Check sheet for the modelled part. Datum: model origin and axes. Units: mm. A direction names the side the tool comes from. Round coordinates to 2 decimals unless told otherwise and drop trailing zeros. Write each loop counter-clockwise with the first axis right and the second up, starting at its lowest first coordinate (ties: lowest second). Pieces come first, ordered by that corner, then holes. Notation, with made-up numbers: (-25.75, 3) -> (31.25, 3) arc R18 ccw to (31.25, 8) -> close; hole circle Ø6 at (53.5, 32). An arc over 180 degrees is marked (long way). Use one line per item in the form item = value. Start each with the question number.
```python
from build123d import *

# Parameters (mm, degrees)
F2_R = 2


with BuildPart() as f1:
    # F0 (on Right) → F1 (revolve)
    with BuildSketch(Plane.YZ):
        Polygon((0, 22), (0, 6), (48.5, 6), (48.5, 15), (48, 15), (48, 30), (8.5, 30), (8.5, 18), (6.5, 18), (6.5, 22), align=None)
    revolve(axis=Axis((0, 19.820221, 0), (0, 1, 0)))

    # F2
    f2_edges = [f1.edges().sort_by_distance(p)[0] for p in [
        (0, 0, -22),
        (0, 8.5, -30),
        (0, 48, -30),
    ]]
    fillet(f2_edges, radius=F2_R)


solid = f1.part
```
1. Sectioned sample at B-B (z = 0). Enter the section's corners in (x, y).
2. Scan lines: probe 1 along Y at (x, z) = (-5.5, -18); probe 2 along X at (y, z) = (36, 0); probe 3 along Y at (x, z) = (23, -13). Record each from-to range of solid material in increasing order.
3. Sectioned sample at A-A (x = 0). Enter the section's corners in (y, z).
4. Depth check by flat-ended pin: pin 1 (4 mm diameter, centred on y = 12.5, z = 15, fed in from +X); pin 2 (3 mm diameter, centred on x = 10, y = 40, fed in from -Z); pin 3 (2 mm diameter, centred on y = 8, z = 19, fed in from +X). Enter the tip coordinate at first touch or a pass-through.
5. Mould release check, pull along Y, two halves, no side actions. Record for faces 1 (the face through (-6.5, 48.5, 0.2)), 2 (the face through (-16.2, 6.5, 8.3)), 3 (the face through (-21.477, 4.219, -4.769)): +Y half, -Y half, draft (parallel to the pull), parting line (faces both ways), or undercut.
6. Sectioned sample at C-C (y = 29). Enter the section's corners in (x, z), and give its area (3 significant figures).
7. Tool access check on faces 4 (the face through (0, 25, -6)), 5 (the face through (0.66, 48.246, -14.985)), 6 (the face through (17.847, 7.486, -2.343)). Record the directions out of +Z, -Z, +X, -X, +Y, -Y that give a thin tool (end or side, any length) a straight path to the whole face; none if there is none.
Returned:
q1.outline = (-30, 10.5) arc R2 ccw to (-28, 8.5) -> (-18, 8.5) -> (-18, 6.5) -> (-22, 6.5) -> (-22, 2) arc R2 ccw to (-20, 0) -> (-6, 0) -> (-6, 48.5) -> (-15, 48.5) -> (-15, 48) -> (-28, 48) arc R2 ccw to (-30, 46) -> close; (6, 0) -> (20, 0) arc R2 ccw to (22, 2) -> (22, 6.5) -> (18, 6.5) -> (18, 8.5) -> (28, 8.5) arc R2 ccw to (30, 10.5) -> (30, 46) arc R2 ccw to (28, 48) -> (15, 48) -> (15, 48.5) -> (6, 48.5) -> close
q2.probe_1 = 0 to 6.5, 8.5 to 48
q2.probe_2 = -30 to -6, 6 to 30
q2.probe_3 = 8.5 to 48
q3.outline = (0, -20) arc R2 ccw to (2, -22) -> (6.5, -22) -> (6.5, -18) -> (8.5, -18) -> (8.5, -28) arc R2 ccw to (10.5, -30) -> (46, -30) arc R2 ccw to (48, -28) -> (48, -15) -> (48.5, -15) -> (48.5, -6) -> (0, -6) -> close; (0, 6) -> (48.5, 6) -> (48.5, 15) -> (48, 15) -> (48, 28) arc R2 ccw to (46, 30) -> (10.5, 30) arc R2 ccw to (8.5, 28) -> (8.5, 18) -> (6.5, 18) -> (6.5, 22) -> (2, 22) arc R2 ccw to (0, 20) -> close
q4.pin_1 = 27.04
q4.pin_2 = -28.77
q4.pin_3 = 22.54
q5.face_1 = +Y half
q5.face_2 = undercut
q5.face_3 = draft
q6.outline = circle Ø60 at (0, 0); hole circle Ø12 at (0, 0)
q6.area = 2,710 mm^2
q7.face_4 = +Y, -Y
q7.face_5 = +Y
q7.face_6 = none
